```python
from build123d import *

# Parameters (mm, degrees)
SKETCH1_W           = 100.75
SKETCH1_H           = 94
SKETCH1_R           = 4
SKETCH1_R_2         = 0.75
BOSS_EXTRUDE1_DEPTH = 14
SKETCH2_W           = 96.749994904
SKETCH2_H           = 90.000003576
CUT_EXTRUDE1_DEPTH  = 12
SKETCH3_R           = 3.548963513
SKETCH3_R_2         = 3.408819902
SKETCH3_R_3         = 3.5
BOSS_EXTRUDE2_DEPTH = 6.3
SKETCH4_R           = 4
BOSS_EXTRUDE3_DEPTH = 6.3
SKETCH7_R           = 1.5
CUT_EXTRUDE2_DEPTH  = 10
SKETCH11_R          = 3
CUT_EXTRUDE3_DEPTH  = 10
SKETCH10_R          = 1.5
CUT_EXTRUDE4_DEPTH  = 10
SKETCH9_R           = 1.5
CUT_EXTRUDE5_DEPTH  = 10
SKETCH12_W          = 79
SKETCH12_H          = 51.75
CUT_EXTRUDE6_DEPTH  = 6.3
FILLET1_R           = 4
SKETCH13_W          = 1
SKETCH13_H          = 24
CUT_EXTRUDE7_DEPTH  = 3


with BuildPart() as part:
    # Sketch1 → Boss-Extrude1 (new body)
    with BuildSketch(Plane.XY):
        with Locations((5.613095238, -11.055404346)):
            Rectangle(SKETCH1_W, SKETCH1_H)
        with Locations((42.159546405, -46.524709499)):
            Circle(SKETCH1_R, mode=Mode.SUBTRACT)
        with Locations((18.44753625, -46.478480461)):
            Circle(SKETCH1_R_2, mode=Mode.SUBTRACT)
        with Locations((19.234631499, -43.590885312)):
            Circle(SKETCH1_R_2, mode=Mode.SUBTRACT)
        with Locations((21.306759983, -41.506641185)):
            Circle(SKETCH1_R_2, mode=Mode.SUBTRACT)
        with Locations((24.200000332, -40.756641185)):
            Circle(SKETCH1_R_2, mode=Mode.SUBTRACT)
        with Locations((27.10075415, -41.594119124)):
            Circle(SKETCH1_R_2, mode=Mode.SUBTRACT)
        with Locations((29.079295953, -43.730354454)):
            Circle(SKETCH1_R_2, mode=Mode.SUBTRACT)
        with Locations((26.35075415, -43.930808011)):
            Circle(SKETCH1_R_2, mode=Mode.SUBTRACT)
        with Locations((24.200000332, -43.085140439)):
            Circle(SKETCH1_R_2, mode=Mode.SUBTRACT)
        with Locations((22.056759983, -43.930808011)):
            Circle(SKETCH1_R_2, mode=Mode.SUBTRACT)
        with Locations((20.829643134, -45.984414142)):
            Circle(SKETCH1_R_2, mode=Mode.SUBTRACT)
        with Locations((21.208891166, -48.100122201)):
            Circle(SKETCH1_R_2, mode=Mode.SUBTRACT)
        with Locations((23.009299731, -49.814525249)):
            Circle(SKETCH1_R_2, mode=Mode.SUBTRACT)
        with Locations((25.331945715, -49.660785564)):
            Circle(SKETCH1_R_2, mode=Mode.SUBTRACT)
        with Locations((27.10075415, -48.100122201)):
            Circle(SKETCH1_R_2, mode=Mode.SUBTRACT)
        with Locations((27.425643307, -45.898634663)):
            Circle(SKETCH1_R_2, mode=Mode.SUBTRACT)
        with Locations((29.829295953, -46.454612718)):
            Circle(SKETCH1_R_2, mode=Mode.SUBTRACT)
        with Locations((29.201955135, -49.487574185)):
            Circle(SKETCH1_R_2, mode=Mode.SUBTRACT)
        with Locations((26.912976345, -51.413900689)):
            Circle(SKETCH1_R_2, mode=Mode.SUBTRACT)
        with Locations((23.949532439, -52.163900689)):
            Circle(SKETCH1_R_2, mode=Mode.SUBTRACT)
        with Locations((21.208891166, -51.413900689)):
            Circle(SKETCH1_R_2, mode=Mode.SUBTRACT)
        with Locations((19.234631499, -49.282190221)):
            Circle(SKETCH1_R_2, mode=Mode.SUBTRACT)
        with BuildLine():
            Line((-18.905494332, -35.031726566), (-8.405494332, -35.031726566))
            ThreePointArc((-8.405494332, -35.031726566), (-7.350829628, -36.08639127), (-8.405494332, -37.141055974))
            Line((-8.405494332, -37.141055974), (-18.905494332, -37.141055974))
            ThreePointArc((-18.905494332, -37.141055974), (-19.960159036, -36.08639127), (-18.905494332, -35.031726566))
        make_face(mode=Mode.SUBTRACT)
        with BuildLine():
            Line((-18.905494332, -39.000402281), (-8.405494332, -39.000402281))
            ThreePointArc((-8.405494332, -39.000402281), (-7.412807684, -39.993088929), (-8.405494332, -40.985775577))
            Line((-8.405494332, -40.985775577), (-18.905494332, -40.985775577))
            ThreePointArc((-18.905494332, -40.985775577), (-19.89818098, -39.993088929), (-18.905494332, -39.000402281))
        make_face(mode=Mode.SUBTRACT)
        with BuildLine():
            Line((-18.905494332, -43.093266368), (-8.405494332, -43.093266368))
            ThreePointArc((-8.405494332, -43.093266368), (-7.500570206, -43.998190495), (-8.405494332, -44.903114621))
            Line((-8.405494332, -44.903114621), (-18.905494332, -44.903114621))
            ThreePointArc((-18.905494332, -44.903114621), (-19.810418459, -43.998190495), (-18.905494332, -43.093266368))
        make_face(mode=Mode.SUBTRACT)
    extrude(amount=BOSS_EXTRUDE1_DEPTH)

    # Sketch2 → Cut-Extrude1 (cut)
    with BuildSketch(Plane(origin=(0, 0, 0), x_dir=(-1, 0, 0), z_dir=(0, 0, -1))):
        with Locations((-5.613093018, -11.047617438)):
            Rectangle(SKETCH2_W, SKETCH2_H)
    extrude(amount=-CUT_EXTRUDE1_DEPTH, mode=Mode.SUBTRACT)

    # Sketch3 → Boss-Extrude2 (add)
    with BuildSketch(Plane(origin=(0, 0, 12), x_dir=(-1, 0, 0), z_dir=(0, 0, -1))):
        with Locations((-49.488095238, 29.944595654)):
            Circle(SKETCH3_R)
        with Locations((38.261904762, 29.944595654)):
            Circle(SKETCH3_R_2)
        with Locations((38.261904762, -35.055404346)):
            Circle(SKETCH3_R_3)
        with Locations((-49.488095238, -35.055404346)):
            Circle(SKETCH3_R_3)
    extrude(amount=BOSS_EXTRUDE2_DEPTH)

    # Sketch4 → Boss-Extrude3 (add)
    with BuildSketch(Plane(origin=(0, 0, 12), x_dir=(-1, 0, 0), z_dir=(0, 0, -1))):
        with Locations((-9.238095238, -46.305404346)):
            Circle(SKETCH4_R)
    extrude(amount=BOSS_EXTRUDE3_DEPTH)

    # Sketch7 → Cut-Extrude2 (cut)
    with BuildSketch(Plane(origin=(0, 0, 5.7), x_dir=(-1, 0, 0), z_dir=(0, 0, -1))):
        with Locations((-49.68373898, 29.928867)):
            Circle(SKETCH7_R)
    extrude(amount=-CUT_EXTRUDE2_DEPTH, mode=Mode.SUBTRACT)

    # Sketch11 → Cut-Extrude3 (cut)
    with BuildSketch(Plane(origin=(0, 0, 5.7), x_dir=(-1, 0, 0), z_dir=(0, 0, -1))):
        with Locations((-9.238095238, -46.305404346)):
            Circle(SKETCH11_R)
    extrude(amount=-CUT_EXTRUDE3_DEPTH, mode=Mode.SUBTRACT)

    # Sketch10 → Cut-Extrude4 (cut)
    with BuildSketch(Plane(origin=(0, 0, 5.7), x_dir=(-1, 0, 0), z_dir=(0, 0, -1))):
        with Locations((-49.686899023, -35.059761001)):
            Circle(SKETCH10_R)
    extrude(amount=-CUT_EXTRUDE4_DEPTH, mode=Mode.SUBTRACT)

    # Sketch9 → Cut-Extrude5 (cut)
    with BuildSketch(Plane(origin=(0, 0, 5.7), x_dir=(-1, 0, 0), z_dir=(0, 0, -1))):
        with Locations((38.261904762, 29.944595654)):
            Circle(SKETCH9_R)
        with Locations((38.261904762, -35.055404346)):
            Circle(SKETCH9_R)
    extrude(amount=-CUT_EXTRUDE5_DEPTH, mode=Mode.SUBTRACT)

    # Sketch12 → Cut-Extrude6 (cut)
    with BuildSketch(Plane(origin=(0, 0, 12), x_dir=(-1, 0, 0), z_dir=(0, 0, -1))):
        with Locations((-5.988095238, -2.630404346)):
            Rectangle(SKETCH12_W, SKETCH12_H)
    extrude(amount=-CUT_EXTRUDE6_DEPTH, mode=Mode.SUBTRACT)

    # Fillet1
    fillet1_edges = [part.edges().sort_by_distance(p)[0] for p in [
        (-44.761904762, 35.944595654, 7),
        (55.988095238, 35.944595654, 7),
        (55.988095238, -58.055404346, 7),
        (-44.761904762, -58.055404346, 7),
    ]]
    fillet(fillet1_edges, radius=FILLET1_R)

    # Sketch13 → Cut-Extrude7 (cut)
    with BuildSketch(Plane.ZY.offset(44.761904762)):
        with Locations((0.5, -3.305404346)):
            Rectangle(SKETCH13_W, SKETCH13_H)
    extrude(amount=-CUT_EXTRUDE7_DEPTH, mode=Mode.SUBTRACT)


solid = part.part
```
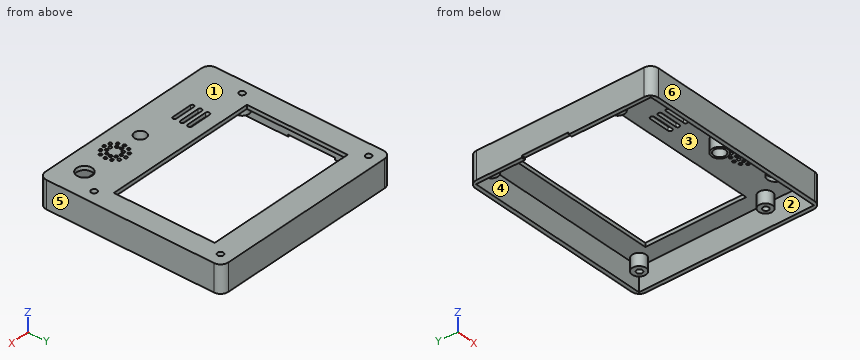
Work out the finished part from the listing and answer in its coordinate system (mm). Face numbers are marked on the shaded views. A direction names the side the tool comes from. Round coordinates to 2 decimals unless told otherwise and drop trailing zeros. Loops run counter-clockwise (first coordinate to the right, second up) from the corner with the lowest first, then second, coordinate; pieces in that order, holes last. Notation, with made-up numbers: (50.25, 24) -> (108.25, 24) arc R10 ccw to (108.25, 38) -> close; hole circle Ø2 at (-20, 78.5). An arc over 180 degrees is marked (long way). Write each question's results on one line, items separated by ' | '. Start each with the question number.
1. Section B-B (y = 13.5) is taken. Determine the outline of the cut face in (x, z), plus the area to 3 significant figures.
2. A tool of negligible diameter and unlimited length cuts with its end or side. For the marked faces 1 and 2, from which of +Z, -Z, +X, -X, +Y, -Y can it reach the whole face along a straight path? Write none if from no direction.
3. Section D-D (x = 32) is taken. Determine the outline of the cut face in (y, z).
4. Find the intervals of material crossed by probe 1 along Y at (x, z) = (22, 5); probe 2 along X at (y, z) = (1, 12.75); probe 3 along X at (y, z) = (-54, 4), in increasing order. Write a range as from..to.
5. Given pin 1 Ø5 at (x, y) = (42, 9) entering from -Z; pin 2 Ø1.6 at (x, y) = (-43.5, -8) entering from -Z; pin 3 Ø3.5 at (x, y) = (-38.26, 29.94) entering from -Z; pin 4 Ø2 at (x, y) = (21.21, -51.41) entering from -Z, each flat-ended and moving along its own axis, determine where each tip first touches the part or whether it passes through.
6. Section C-C (z = 9.75) is taken. State how many separate pieces and enclosed holes the cut face has, plus the area to 3 significant figures.
7. For a pull along X with two mould halves and no side action, classify the marked faces 3, 4, 5 and 6 as +X half, -X half, draft (parallel to the pull), parting line (faces both ways), or undercut.
8. Section A-A (x = -17) is taken. Determine the outline of the cut face in (y, z).
Evaluation:
1) outline: (-44.76, 0) -> (-42.76, 0) -> (-42.76, 12) -> (-33.51, 12) -> (-33.51, 14) -> (-44.76, 14) -> close; (45.49, 12) -> (53.99, 12) -> (53.99, 0) -> (55.99, 0) -> (55.99, 14) -> (45.49, 14) -> close | area: 91.5 mm2
2) face 1: +Z, +X, -X, +Y, -Y | face 2: -Z
3) outline: (-58.06, 0) -> (-56.05, 0) -> (-56.05, 12) -> (-28.51, 12) -> (-28.51, 14) -> (-58.06, 14) -> close; (23.24, 12) -> (33.95, 12) -> (33.95, 0) -> (35.94, 0) -> (35.94, 14) -> (23.24, 14) -> close
4) probe 1: y = -58.06..-56.05, 33.95..35.94 | probe 2: x = -44.76..-33.51, 45.49..55.99 | probe 3: x = -44.76..-42.76, 53.99..55.99
5) pin 1: passes through | pin 2: stops at z = 1 | pin 3: stops at z = 5.7 | pin 4: stops at z = 12
6) separate pieces: 6 | enclosed holes: 6 | area: 896 mm2
7) face 3: undercut | face 4: undercut | face 5: +X half | face 6: draft
8) outline: (-58.06, 0) -> (-56.05, 0) -> (-56.05, 12) -> (-44.9, 12) -> (-44.9, 14) -> (-58.06, 14) -> close; (-43.09, 12) -> (-40.99, 12) -> (-40.99, 14) -> (-43.09, 14) -> close; (-39, 12) -> (-37.14, 12) -> (-37.14, 14) -> (-39, 14) -> close; (-35.03, 12) -> (-28.51, 12) -> (-28.51, 14) -> (-35.03, 14) -> close; (23.24, 12) -> (33.95, 12) -> (33.95, 0) -> (35.94, 0) -> (35.94, 14) -> (23.24, 14) -> close
